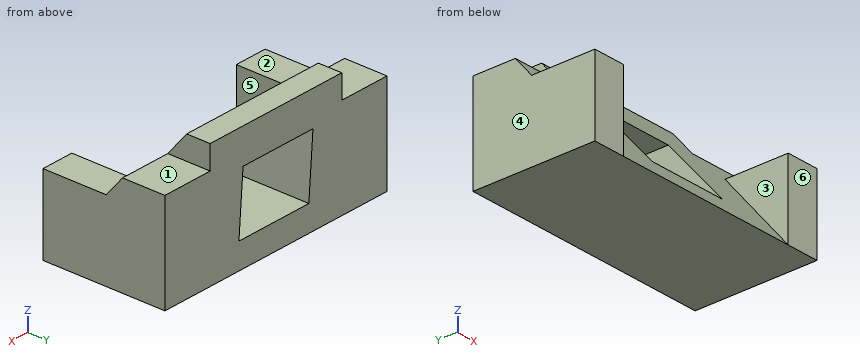
```python
from build123d import *

# Parameters (mm, degrees)
F0_W     = 54
F0_H     = 26
F1_DEPTH = 26
F3_DEPTH = 72.1
F4_W     = 7
F4_H     = 16.7
F5_DEPTH = 26
F6_W     = 11
F6_H     = 5
F7_DEPTH = 25


with BuildPart() as f1:
    # F0 (on Front) → F1 (new body)
    with BuildSketch(Plane.XZ):
        Rectangle(F0_W, F0_H)
    extrude(amount=F1_DEPTH)

    # F2 (on face) → F3 (cut)
    with BuildSketch(Plane.YZ.offset(27)):
        Polygon((-26, -13), (-5, 13), (-26, 13), align=None)
    extrude(amount=-F3_DEPTH, mode=Mode.SUBTRACT)

    # F4 (on face) → F5 (join)
    with BuildSketch(Plane(origin=(0, 0, 0), x_dir=(-1, 0, 0), z_dir=(0, 1, 0))):
        with Locations((-23.5, -4.65)):
            Rectangle(F4_W, F4_H)
        with Locations((23.5, -4.65)):
            Rectangle(F4_W, F4_H)
    extrude(amount=-F5_DEPTH)

    # F6 (on face) → F7 (cut)
    with BuildSketch(Plane(origin=(0, 0, 0), x_dir=(-1, 0, 0), z_dir=(0, 1, 0))):
        with Locations((-21.5, 10.5)):
            Rectangle(F6_W, F6_H)
        with Locations((21.5, 10.5)):
            Rectangle(F6_W, F6_H)
    extrude(amount=-F7_DEPTH, mode=Mode.SUBTRACT)

    # F8 (on face) → F10 section 0
    with BuildSketch(Plane(origin=(0, -9.3804834378, 7.5765443151), x_dir=(1, 0, 0), z_dir=(0, -0.7779411802, 0.6283371071))):
        Polygon((-8, -19.4500001269), (9, -19.4500001269), (8, -2.4794373784), (-9, -2.4794373784), align=None)
    # F9 (on face) → F10 section 1
    with BuildSketch(Plane(origin=(0, 0, 0), x_dir=(-1, 0, 0), z_dir=(0, 1, 0))):
        Polygon((9, 5.6476878747), (-8, 5.6476878747), (-9, -7.5544117386), (8, -7.5544117386), align=None)
    loft(mode=Mode.SUBTRACT)


solid = f1.part
```
Part model, mm, in its own coordinate system. Face numbers are marked on the shaded views. A direction names the side the tool comes from. Round coordinates to 2 decimals unless told otherwise and drop trailing zeros. Write each loop counter-clockwise with the first axis right and the second up, starting at its lowest first coordinate (ties: lowest second). Pieces come first, ordered by that corner, then holes.
Item 1: Probe L1, parallel to X at y = -9.5, z = 5.5; L2, parallel to X at y = -3, z = 11.5; L3, parallel to X at y = -6, z = 4. List the from-to ranges inside material, lowest first.
Results:
L1: x = -27 to -8.99, 8.01 to 27
L2: x = -16 to 16
L3: x = -27 to -8.88, 8.12 to 27
Item 2: Cut at C-C, the plane x = -19. Give the cut face in (y, z), plus the area to 3 significant figures.
Results:
outline: (-26, -13) - (0, -13) - (0, 8) - (-9.04, 8) - close
area: 368 mm2
Item 3: Cut at A-A, the plane x = -3. Give the cut face in (y, z).
Results:
outline: (-26, -13) - (0, -13) - (0, -7.55) - (-21.6, -7.55) - close; (-10.94, 5.65) - (0, 5.65) - (0, 13) - (-5, 13) - close
Item 4: Two-plate mould, pull along X, no slides. Class the marked faces 4, 5 and 6: +X half, -X half, draft (parallel to the pull), parting line (faces both ways), or undercut.
Results:
face 4: -X half
face 5: undercut
face 6: draft
Item 5: Which spindle directions (+Z, -Z, +X, -X, +Y, -Y) get a long thin tool onto all of the face, cutting with end or side? Do the marked faces 1, 2 and 3. Say none if no direction does.
Results:
face 1: +Z, +X, +Y, -Y
face 2: +Z, +X, -X, -Y
face 3: +Z, -Y
Item 6: Cut at B-B, the plane z = -9. Give the cut face in (x, y).
Results:
outline: (-27, -26) - (-20, -26) - (-20, -22.77) - (20, -22.77) - (20, -26) - (27, -26) - (27, 0) - (-27, 0) - close
Item 7: Drop flat-ended pins along their axis: pin 1 Ø7 at (x, y) = (21.5, -3.5) entering from +Z; pin 2 Ø5.5 at (x, y) = (22, -18.5) entering from +Z; pin 3 Ø4 at (y, z) = (-4, 10.5) entering from -X. Give the stop position or say it passes through.
Results:
pin 1: stops at z = 8
pin 2: stops at z = 3.7
pin 3: stops at x = -16
Item 8: Cut at D-D, the plane z = 11.75. Give the cut face in (x, y).
Results:
outline: (-16, -6.01) - (16, -6.01) - (16, 0) - (-16, 0) - close
